```python
from build123d import *

# Parameters (mm, degrees)
F1_DEPTH = 6


# Not quite as in the source:
# - ends of sketch curves that miss each other by under 0.0002 mm in the source are joined


with BuildPart() as f1:
    # F0 (on Front) → F1 (new body)
    with BuildSketch(Plane.XZ):
        with BuildLine():
            ThreePointArc((50.6578879007, 28.8518228186), (0, 41.809787), (-50.6578879007, 28.8518228186))
            Line((-50.6578879007, 28.8518228186), (-9.861388, -41.809787))
            ThreePointArc((-9.861388, -41.809787), (4.558e-07, -39.690213), (9.8613887008, -41.8097876638))
            Line((9.8613887008, -41.8097876638), (50.6578879007, 28.8518228186))
        make_face()
        with BuildLine():
            ThreePointArc((10.3923048841, -12.0902129331), (0, -18.090213), (-10.3923048841, -12.0902129331))
            Line((-10.3923048841, -12.0902129331), (-22.500773, 8.88227))
            ThreePointArc((-22.500773, 8.88227), (-22.9286788819, 20.0710113186), (-13.93616106, 26.7422673895))
            ThreePointArc((-13.93616106, 26.7422673895), (4.942e-07, 27.809787), (13.9361619582, 26.7422667287))
            ThreePointArc((13.9361619582, 26.7422667287), (22.92867999, 20.0710110932), (22.5007736341, 8.8822696339))
            Line((22.5007736341, 8.8822696339), (10.3923048841, -12.0902129331))
        make_face(mode=Mode.SUBTRACT)
    extrude(amount=F1_DEPTH)


solid = f1.part
```
Model file for the job. Use its own axes, mm. A direction names the side the tool comes from. Round coordinates to 2 decimals unless told otherwise and drop trailing zeros. Write each loop counter-clockwise with the first axis right and the second up, starting at its lowest first coordinate (ties: lowest second). Pieces come first, ordered by that corner, then holes. Notation, with made-up numbers: M 82.25,-31 L 124.25,-31 A6 ccw 124.25,-25 Z; hole C 19.25,75.5 d3. An arc over 180 degrees is marked long. Put each result on its own line as item: value.
Item 1: Cut at A-A (y = -3.9). List the corners of the cut face in (x, z), and give its area (3 significant figures).
Responses:
outline: M -50.66,28.85 L -9.86,-41.81 A24 cw 9.86,-41.81 L 50.66,28.85 A105.5 ccw Z; hole M -22.5,8.88 L -10.39,-12.09 A12 ccw 10.39,-12.09 L 22.5,8.88 A12 ccw 13.94,26.74 A91.5 ccw -13.94,26.74 A12 ccw Z
area: 3,540 mm²
Item 2: Probe L1, parallel to X at y = -5.3, z = -16; L2, parallel to X at y = -2.9, z = -13; L3, parallel to Z at x = 12.5, y = -4. List the from-to ranges inside material, lowest first. Write a range as from..to.
Responses:
L1: -24.76..-6.77, 6.77..24.76
L2: -26.49..-9.81, 9.81..26.49
L3: -37.24..-8.44, 26.95..41.07
Item 3: Cut at B-B (x = 4.5). List the corners of the cut face in (y, z), and give its area (3 significant figures).
Responses:
outline: M -6,-40.12 L 0,-40.12 L 0,-17.21 L -6,-17.21 Z; M -6,27.7 L 0,27.7 L 0,41.71 L -6,41.71 Z
area: 221 mm²
Item 4: Tool access for faces 4 (the cylindrical face through (0.74, -2.958, 41.807)), 5 (the cylindrical face through (0.18, -2.96, -18.09)): list every direction of +Z, -Z, +X, -X, +Y, -Y with a clear straight run to the whole face (end or side of a thin tool).
Responses:
face 4: +Z, +Y, -Y
face 5: +Y, -Y
Item 5: Cut at C-C (z = 4). List the corners of the cut face in (x, y).
Responses:
outline: M -36.31,-6 L -19.68,-6 L -19.68,0 L -36.31,0 Z; M 19.68,-6 L 36.31,-6 L 36.31,0 L 19.68,0 Z
Item 6: Flat gauge pins, fed straight in: P1, Ø1.5, axis at x = -16.5, y = -4, coming from the -Z side; P2, Ø1, axis at x = -36.5, y = -5.5, coming from the -Z side. Where does each tip first touch, or does it go through?
Responses:
P1: z = -31.61
P2: z = 3.46
Item 7: Cut at D-D (x = -26). List the corners of the cut face in (y, z), and give its area (3 significant figures).
Responses:
outline: M -6,-13.86 L 0,-13.86 L 0,38.56 L -6,38.56 Z
area: 314 mm²
Item 8: Mould opens along X. For faces 1 (the flat face through (-30.55, -2.96, -5.98)), 2 (the cylindrical face through (-0.2, -2.96, 27.81)), 3 (the flat face through (29.974, -2.958, -6.974)) say: +X half, -X half, draft (parallel to the pull), parting line (faces both ways), or undercut.
Responses:
face 1: -X half
face 2: undercut
face 3: +X half
